Can you work these out from the model? Positions are in its coordinate system, mm. A direction names the side the tool comes from. Give positions to 0.01 mm unless a question says otherwise; leave off trailing zeros. Order: outer loops, then holes, each group sorted by start corner. A loop starts at its lowest first (then second) coordinate and runs counter-clockwise, first axis right, second up. Notation, with made-up numbers: M 89,46.25 L 113,46.25 A29 ccw 113,71.25 Z; hole C 2,23.5 d4. An arc over 180 degrees is marked long. Use a Markdown table: item, result. Add a question column.
from build123d import *

# Parameters (mm, degrees)
SKETCH1_W           = 100
SKETCH1_H           = 14
SKETCH1_R           = 1.7
BOSS_EXTRUDE1_DEPTH = 15
SKETCH3_R           = 1.7
CUT_EXTRUDE2_DEPTH  = 55.046276467
CUT_EXTRUDE3_START  = -7
CUT_EXTRUDE3_DEPTH  = 1.5
CUT_EXTRUDE4_DEPTH  = 6
FILLET4_R           = 3
CUT_EXTRUDE5_DEPTH  = 13.6


with BuildPart() as part:
    # Sketch1 → Boss-Extrude1 (new body)
    with BuildSketch(Plane(origin=(0, 0, 0), x_dir=(1, 0, 0), z_dir=(0, 1, 0))):
        Rectangle(SKETCH1_W, SKETCH1_H)
        with Locations(Location((-27.175, 2, 0), (0, 0, 270))):
            Circle(SKETCH1_R, mode=Mode.SUBTRACT)
        with Locations(Location((27.175, 2, 0), (0, 0, 270))):
            Circle(SKETCH1_R, mode=Mode.SUBTRACT)
    extrude(amount=BOSS_EXTRUDE1_DEPTH)

    # Sketch3 → Cut-Extrude2 (cut, through all)
    with BuildSketch(Plane.XY.offset(7)):
        with Locations((-42, 9)):
            Circle(SKETCH3_R)
        with Locations((42, 9)):
            Circle(SKETCH3_R)
    extrude(amount=-CUT_EXTRUDE2_DEPTH, mode=Mode.SUBTRACT)

    # Sketch4 → Cut-Extrude3 (cut, symmetric)
    with BuildSketch(Plane.XY.offset(7).offset(CUT_EXTRUDE3_START)):
        Polygon((-45, 10.732050808), (-45, 16.451909609), (-39, 16.451909609), (-39, 10.732050808), (-39, 7.267949192), (-42, 5.535898385), (-45, 7.267949192), align=None)
        Polygon((39, 16.451909609), (39, 10.732050808), (39, 7.267949192), (42, 5.535898385), (45, 7.267949192), (45, 10.732050808), (45, 16.451909609), align=None)
    extrude(amount=CUT_EXTRUDE3_DEPTH, both=True, mode=Mode.SUBTRACT)

    # Sketch5 → Cut-Extrude4 (cut)
    with BuildSketch(Plane(origin=(0, 15, 0), x_dir=(1, 0, 0), z_dir=(0, 1, 0))):
        Polygon((25.442949192, -1), (23.710898385, 2), (25.442949192, 5), (28.907050808, 5), (30.639101615, 2), (28.907050808, -1), align=None)
    extrude(amount=-CUT_EXTRUDE4_DEPTH, mode=Mode.SUBTRACT)

    # Fillet4
    fillet4_edges = [part.edges().sort_by_distance(p)[0] for p in [
        (50, 7.5, 7),
        (-50, 7.5, 7),
        (-50, 7.5, -7),
        (50, 7.5, -7),
    ]]
    fillet(fillet4_edges, radius=FILLET4_R)

    # Sketch6 → Cut-Extrude5 (cut)
    with BuildSketch(Plane(origin=(0, 15, 0), x_dir=(1, 0, 0), z_dir=(0, 1, 0))):
        Polygon((-35, -7), (-41.338104143, 7), (-21.338104143, 7), (-15, -7), align=None)
    extrude(amount=-CUT_EXTRUDE5_DEPTH, mode=Mode.SUBTRACT)


solid = part.part
1. If we section it at A-A, the plane y = 13.25: List the corners of the cut face in (x, z) for me, then the cut area to 3 significant figures.
2. I need wall thicknesses on L1, parallel to Z at x = -44.5, y = 13; L2, parallel to X at y = 10, z = -1.25; L3, parallel to X at y = 8.25, z = 5. Which ranges of each line are inside material? Lowest first, please. Write a range as [from, to].
3. We'd pull the mould along Z, two halves only. Please class faces 4 (the face through (-18.213, 8.295, -0.098)), 5 (the face through (27, 12, 1)), 6 (the face through (-43.35, 7.97, 4.29)): +Z half, -Z half, draft (parallel to the pull), parting line (faces both ways), or undercut.
4. Will these pins go through, and if not, where does the flat tip stop? pin 1 (6 mm diameter, centred on x = -25.5, z = -2, fed in from -Y); pin 2 (4 mm diameter, centred on x = -27.175, z = -2, fed in from +Y); pin 3 (2 mm diameter, centred on x = 42, y = 9, fed in from -Z); pin 4 (3 mm diameter, centred on x = 28, z = -1.5, fed in from +Y).
5. On a 3-axis mill with a long thin cutter (end or side, diameter ignored), from which of +Z, -Z, +X, -X, +Y, -Y can I reach the whole of each face in a straight line? I mean faces 1 (the face through (-45, 11, 0)), 2 (the face through (50, 7, 0)), 3 (the face through (-38.125, 8.295, 0.098)). Say none if no direction works.
6. If we section it at B-B, the plane x = -23.5: List the corners of the cut face in (y, z) for me.
Geometry results:
| question | item | result |
|---|---|---|
| 1 | outline | M -50,-4 A3 ccw -47,-7 L -41.34,-7 L -35,7 L -47,7 A3 ccw -50,4 Z; M -21.34,-7 L 47,-7 A3 ccw 50,-4 L 50,4 A3 ccw 47,7 L -15,7 Z; hole M -45,-1.5 L -39,-1.5 L -39,1.5 L -45,1.5 Z; hole M 23.71,-2 L 25.44,-5 L 28.91,-5 L 30.64,-2 L 28.91,1 L 25.44,1 Z; hole M 39,-1.5 L 45,-1.5 L 45,1.5 L 39,1.5 Z |
| 1 | area | 1,050 mm^2 |
| 2 | L1 | z = [-7, -1.5], [1.5, 7] |
| 2 | L2 | x = [-50, -45], [-39, -38.73], [-18.73, 24.14], [30.21, 39], [45, 50] |
| 2 | L3 | x = [-49.83, -43.53], [-40.47, -35.91], [-15.91, 40.47], [43.53, 49.83] |
| 3 | face 4 | +Z half |
| 3 | face 5 | undercut |
| 3 | face 6 | draft |
| 4 | pin 1 | stops at y = 0 |
| 4 | pin 2 | stops at y = 1.4 |
| 4 | pin 3 | passes through |
| 4 | pin 4 | stops at y = 9 |
| 5 | face 1 | +Y |
| 5 | face 2 | +Z, -Z, +X, +Y, -Y |
| 5 | face 3 | -Z, +Y |
| 6 | outline | M 0,-7 L 1.4,-7 L 1.4,7 L 0,7 Z |
